Model file for the job. Use its own axes, mm. Face numbers are marked on the shaded views. A direction names the side the tool comes from. Coordinates: 2 decimals unless noted, no trailing zeros. Write each loop counter-clockwise with the first axis right and the second up, starting at its lowest first coordinate (ties: lowest second). Pieces come first, ordered by that corner, then holes. Notation, with made-up numbers: (64, -9) -> (85, -9) arc R10 cw to (85, -4) -> close; hole circle Ø10 at (-32, 47.5). An arc over 180 degrees is marked (long way). Write item = value, one per line. Start each with the question number.
from build123d import *

# Parameters (mm, degrees)
SKETCH3_R = 2.3749


with BuildPart() as part:
    # Sweep1: sweep along a path in Sketch4
    with BuildLine(Plane.XY) as sweep1_path:
        Line((0, 23.0251), (-10.35, 23.0251))
        ThreePointArc((-10.35, 23.0251), (-14.274371925, 21.399571925), (-15.8999, 17.4752))
        Line((-15.8999, 17.4752), (-15.8999, 0))
    # Sketch3 → Sweep1 (sweep)
    with BuildSketch(Plane(origin=(0, 0, 0), x_dir=(1, 0, 0), z_dir=(0, 1, 0))):
        with Locations((-15.8999, 0)):
            Circle(SKETCH3_R)
    sweep(path=sweep1_path.line)

    # Mirror1: part across plane


with BuildPart() as part_1:
    add(part.part)
    add(part.part.mirror(Plane(origin=(0, 0, 0), x_dir=(0, 0, 1), z_dir=(1, 0, 0))))


solid = part_1.part
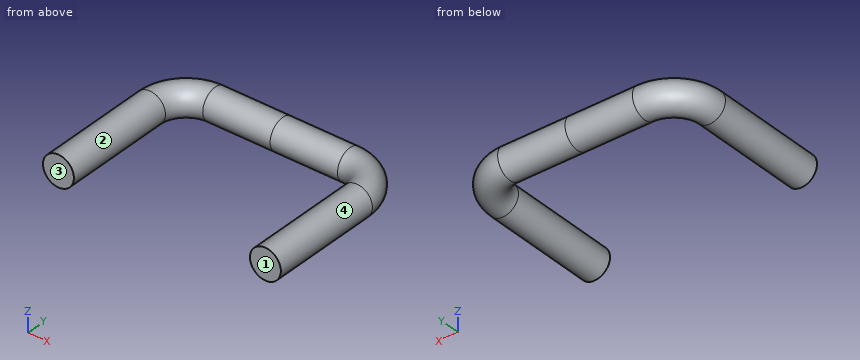
(1) Drop a flat-ended pin along its axis: pin 1 Ø1 at (y, z) = (8.5, -2) entering from -X. Give the stop position or say it passes through.
(2) Saw through at A-A (z = 0). Give the cut face in (x, y) (3 decimals), then the cut area to 3 significant figures.
(3) 3-axis set-ups, long thin cutter, end or side, ignore diameter. For the marked faces 3 and 4: which of +Z, -Z, +X, -X, +Y, -Y reach the whole face in a straight line?
(4) Saw through at D-D (z = 1.8). Give the cut face in (x, y).
(5) Mould opens along X. For the marked faces 1 and 2 say: released by +X, released by -X, zero draft, split by the parting line, or undercut.
(6) Saw through at B-B (y = 7.75). Give the cut face in (x, z) (3 decimals).
(7) Saw through at C-C (x = -8). Give the cut face in (y, z), then the cut area to 3 significant figures.
(8) Drill centre lines: line 1 along X through (y, z) = (9.75, -0.1); line 2 along X through (y, z) = (18.75, 2.15); line 3 along Y through (x, z) = (8, 0.1). Where is each one in solid material? Low to high.
Returned:
q1.pin_1 = -17.74
q2.outline = (-18.275, 0) -> (-13.525, 0) -> (-13.525, 17.475) arc R3.175 cw to (-10.35, 20.65) -> (10.35, 20.65) arc R3.175 cw to (13.525, 17.475) -> (13.525, 0) -> (18.275, 0) -> (18.275, 17.475) arc R7.925 ccw to (10.35, 25.4) -> (-10.35, 25.4) arc R7.925 ccw to (-18.275, 17.475) -> close
q2.area = 347 mm2
q3.face_3 = +Z, -Z, +X, -X, -Y
q3.face_4 = -Y
q4.outline = (-17.45, 0) -> (-14.35, 0) -> (-14.35, 17.48) arc R4 cw to (-10.35, 21.48) -> (10.35, 21.48) arc R4 cw to (14.35, 17.48) -> (14.35, 0) -> (17.45, 0) -> (17.45, 17.48) arc R7.1 ccw to (10.35, 24.57) -> (-10.35, 24.57) arc R7.1 ccw to (-17.45, 17.48) -> close
q5.face_1 = zero draft
q5.face_2 = undercut
q6.outline = circle Ø4.75 at (-15.9, 0); circle Ø4.75 at (15.9, 0)
q7.outline = circle Ø4.75 at (23.03, 0)
q7.area = 17.7 mm2
q8.line_1 = -18.27 to -13.53, 13.53 to 18.27
q8.line_2 = -16.78 to -14.71, 14.71 to 16.78
q8.line_3 = 20.65 to 25.4
